Read the model definition and answer for the solid it produces. Units are mm, in the model's axes. Face numbers are marked on the shaded views. A direction names the side the tool comes from. Give positions to 0.01 mm unless a question says otherwise; leave off trailing zeros. Loops run counter-clockwise (first coordinate to the right, second up) from the corner with the lowest first, then second, coordinate; pieces in that order, holes last. Notation, with made-up numbers: (-36.75, 49) - (-25.75, 49) arc R21 ccw to (-25.75, 53) - close; hole circle Ø11 at (7.25, 89.5). An arc over 180 degrees is marked (long way). Put each result on its own line as item: value. Start each with the question number.
1. Given pin 1 Ø2 at (x, z) = (7, 10) entering from -Y; pin 2 Ø8 at (x, y) = (18, -15.5) entering from -Z, each flat-ended and moving along its own axis, determine where each tip first touches the part or whether it passes through.
2. A cutting plane is placed at B-B, the plane z = 0. Determine the outline of the cut face in (x, y), plus the area to 3 significant figures.
3. A cutting plane is placed at D-D, the plane y = 5.5. Determine the outline of the cut face in (x, z), plus the area to 3 significant figures.
4. A cutting plane is placed at C-C, the plane x = 18. Determine the outline of the cut face in (y, z), plus the area to 3 significant figures.
5. For the marked faces 1 and 2, determine the directions among +Z, -Z, +X, -X, +Y, -Y from which every point of the face is accessible in a straight line to the end or side of a thin tool.
6. Consider L1, parallel to Z at x = 0, y = 4.5; L2, parallel to Y at x = 11, z = 18.5; L3, parallel to X at y = 1.5, z = 11. Determine where each line is inside the solid, lowest interval first. Write a range as from..to.
7. A cutting plane is placed at A-A, the plane x = 0. Determine the outline of the cut face in (y, z).
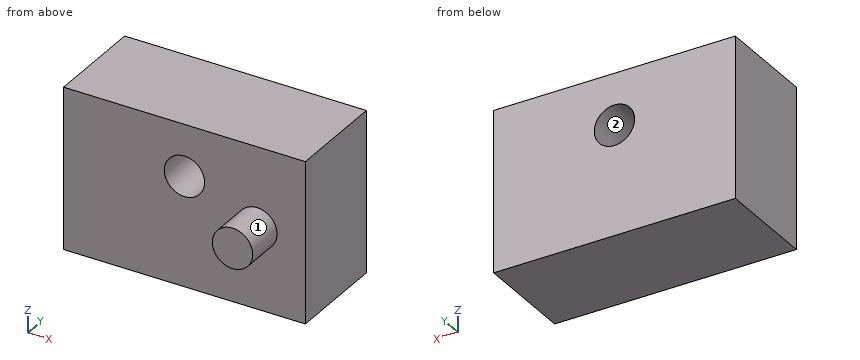
```python
from build123d import *

# Parameters (mm, degrees)
F0_W     = 60
F0_H     = 40
F1_DEPTH = 12.5
F2_R     = 5
F3_DEPTH = 10
F4_R     = 5
F5_DEPTH = 25


# Not quite as in the source:
# - a feature names something its author has since deleted; it is built from what else it names


with BuildPart() as f1:
    # F0 (on Front) → F1 (new body, symmetric)
    with BuildSketch(Plane.XZ):
        Rectangle(F0_W, F0_H)
    extrude(amount=F1_DEPTH, both=True)

    # F2 (on face) → F3 (join)
    with BuildSketch(Plane.XZ.offset(12.5)):
        with Locations((18, 0)):
            Circle(F2_R)
    extrude(amount=F3_DEPTH)

    # F4 (on face) → F5 (cut)
    with BuildSketch(Plane.XZ.offset(12.5)):
        with Locations((0, 7.2016329505)):
            Circle(F4_R)
    extrude(amount=-F5_DEPTH, mode=Mode.SUBTRACT)


solid = f1.part
```
Return value:
1. pin 1: stops at y = -12.5
1. pin 2: stops at z = -20
2. outline: (-30, -12.5) - (13, -12.5) - (13, -22.5) - (23, -22.5) - (23, -12.5) - (30, -12.5) - (30, 12.5) - (-30, 12.5) - close
2. area: 1,600 mm2
3. outline: (-30, -20) - (30, -20) - (30, 20) - (-30, 20) - close; hole circle Ø10 at (0, 7.2)
3. area: 2,320 mm2
4. outline: (-22.5, -5) - (-12.5, -5) - (-12.5, -20) - (12.5, -20) - (12.5, 20) - (-12.5, 20) - (-12.5, 5) - (-22.5, 5) - close
4. area: 1,100 mm2
5. face 1: -Y
5. face 2: +Y, -Y
6. L1: z = -20..2.2, 12.2..20
6. L2: y = -12.5..12.5
6. L3: x = -30..-3.25, 3.25..30
7. outline: (-12.5, -20) - (12.5, -20) - (12.5, 2.2) - (-12.5, 2.2) - close; (-12.5, 12.2) - (12.5, 12.2) - (12.5, 20) - (-12.5, 20) - close
